Work out the finished part from the listing and answer in its coordinate system (mm). Coordinates: 2 decimals unless noted, no trailing zeros. Write each loop counter-clockwise with the first axis right and the second up, starting at its lowest first coordinate (ties: lowest second). Pieces come first, ordered by that corner, then holes. Notation, with made-up numbers: M 2.25,29.5 L 44.25,29.5 A27 cw 44.25,68.5 Z; hole C 56.25,61.25 d2. An arc over 180 degrees is marked long. Answer as CSV lines item,"result". Start each with the question number.
(1) A cutting plane is placed at C-C on z = 1.5. Give the vertices of the cut face in (x, y).
(2) Find the intervals of material crossed by L1, parallel to Y at x = 294.5, z = 3.25; L2, parallel to X at y = 50, z = 1; L3, parallel to Y at x = 176.5, z = 1.5, in increasing order. Write a range as [from, to].
(3) Flat-ended cylindrical pins translate along their axes: P1, Ø1.5, axis at x = 186.5, z = 4.5, coming from the -Y side; P2, Ø2, axis at y = 77, z = 3.5, coming from the +X side; P3, Ø1.5, axis at x = 143, z = 5.5, coming from the +Y side. Find the tip coordinate at first contact, or state that the pin passes through.
from build123d import *

# Parameters (mm, degrees)
BOSS_EXTRUDE1_DEPTH     = 6.35
CHAMFER1_SIZE           = 3.175
CUT_EXTRUDE1_DEPTH      = 421.64
CUT_EXTRUDE1_DEPTH_BACK = 27.432
SKETCH2_R               = 50.8


with BuildPart() as part:
    # Sketch1 → Boss-Extrude1 (new body)
    with BuildSketch(Plane.XY):
        Polygon((279.4, 152.4), (0, 0), (279.4, 0), align=None)
        Polygon((279.4, 152.4), (279.4, 0), (406.4, 0), (381, 152.4), align=None)
    extrude(amount=BOSS_EXTRUDE1_DEPTH)

    # Chamfer1
    chamfer1_edges = [part.edges().sort_by_distance(p)[0] for p in [
        (393.7, 76.2, 6.35),
        (393.7, 76.2, 0),
        (139.7, 76.2, 0),
        (139.7, 76.2, 6.35),
    ]]
    chamfer(chamfer1_edges, length=CHAMFER1_SIZE - 0.0001)  # a hair under: the kernel refuses the full size

    # Sketch2 → Cut-Extrude1 (cut, two sides: drawn at the far end of the back side and taken through both)
    with BuildSketch(Plane(origin=(0, 0, 0), x_dir=(0, 0, -1), z_dir=(1, 0, 0)).offset(-CUT_EXTRUDE1_DEPTH_BACK)):
        with Locations((-3.175, -50.700684167)):
            Circle(SKETCH2_R)
    extrude(amount=CUT_EXTRUDE1_DEPTH + CUT_EXTRUDE1_DEPTH_BACK, mode=Mode.SUBTRACT)


solid = part.part
Here are the results:
1,outline,"M 3.63,0.07 L 404.69,0.07 L 379.3,152.4 L 282.9,152.4 Z"
2,L1,"y = [0.1, 152.4]"
2,L2,"x = [96.21, 395.86]"
2,L3,"y = [0.07, 94.36]"
3,P1,"stops at y = 0.06"
3,P2,"stops at x = 393.72"
3,P3,"stops at y = 76.3"
